from build123d import *

# Parameters (mm, degrees)
SKETCH1_R           = 0.15
SKETCH6_R           = 0.2
BOSS_EXTRUDE1_DEPTH = 0.15


with BuildPart() as part:
    # Sweep1: sweep along a path in Sketch3
    with BuildLine(Plane.XY) as sweep1_path:
        Line((0, 0), (0.05, 0))
        ThreePointArc((0.05, 0), (0.262132034, -0.087867966), (0.35, -0.3))
        Line((0.35, -0.3), (0.35, -30))
    # Sketch1 → Sweep1 (sweep)
    with BuildSketch(Plane(origin=(0, 0, 0), x_dir=(0, 0, -1), z_dir=(1, 0, 0))):
        Circle(SKETCH1_R)
    sweep(path=sweep1_path.line)

    # Sketch6 → Boss-Extrude1 (add)
    with BuildSketch(Plane.ZY):
        Circle(SKETCH6_R)
    extrude(amount=-BOSS_EXTRUDE1_DEPTH)

    # Sketch4 → Revolve2 (revolve)
    with BuildSketch(Plane.ZY):
        with BuildLine():
            Line((0, 0.25), (0, -0.25))
            ThreePointArc((0, -0.25), (-0.25, 0), (0, 0.25))
        make_face()
    revolve(axis=Axis((0, 0.25, 0), (0, -1, 0)))


solid = part.part
Part model, mm, in its own coordinate system. Round coordinates to 2 decimals unless told otherwise and drop trailing zeros. Order: outer loops, then holes, each group sorted by start corner. A loop starts at its lowest first (then second) coordinate and runs counter-clockwise, first axis right, second up. Notation, with made-up numbers: (-38.5, 10.25) -> (15.5, 10.25) arc R27 cw to (15.5, 32.25) -> close; hole circle Ø9 at (18.5, 50.5). An arc over 180 degrees is marked (long way). Put each result on its own line as item: value.
Q1. Band-saw the part on A-A (z = 0). Give the cut face in (x, y), and give its area (3 significant figures).
From the geometry:
outline: (0.16, -0.19) arc R0.15 cw to (0.2, -0.3) -> (0.2, -30) -> (0.5, -30) -> (0.5, -0.3) arc R0.45 ccw to (0.22, 0.12) arc R0.25 ccw (long way) to start
area: 9.19 mm2
Q2. Wall check: line 1 (Z direction, x = 0.35, y = -9); line 2 (Y direction, x = -0.05, z = 0). Give the ranges that are in metal, low to high. Write a range as [from, to].
From the geometry:
line 1: z = [-0.15, 0.15]
line 2: y = [-0.24, 0.24]
Q3. Band-saw the part on B-B (y = -26). Give the cut face in (x, z).
From the geometry:
outline: circle Ø0.3 at (0.35, 0)
